from build123d import *

# Parameters (mm, degrees)
SKETCH1_W           = 133.35
SKETCH1_H           = 101.6
BOSS_EXTRUDE1_DEPTH = 3.175
SKETCH2_W           = 3.175
SKETCH2_H           = 12.192
SKETCH2_W_2         = 19.05
SKETCH2_H_2         = 6.35
BOSS_EXTRUDE2_DEPTH = 3.175
SKETCH3_W           = 19.05
SKETCH3_H           = 6.35
SKETCH3_H_2         = 6.604
CUT_EXTRUDE1_DEPTH  = 91.306287849


with BuildPart() as part:
    # Sketch1 → Boss-Extrude1 (new body)
    with BuildSketch(Plane(origin=(0, 0, 0), x_dir=(1, 0, 0), z_dir=(0, 1, 0))):
        Rectangle(SKETCH1_W, SKETCH1_H)
    extrude(amount=BOSS_EXTRUDE1_DEPTH)

    # Sketch2 → Boss-Extrude2 (add)
    with BuildSketch(Plane(origin=(0, 0, 0), x_dir=(-1, 0, 0), z_dir=(0, -1, 0))):
        with Locations((68.2625, -31.75)):
            Rectangle(SKETCH2_W, SKETCH2_H)
        with Locations((68.2625, -6.35)):
            Rectangle(SKETCH2_W, SKETCH2_H)
        with Locations((68.2625, 19.05)):
            Rectangle(SKETCH2_W, SKETCH2_H)
        with Locations((68.2625, 44.45)):
            Rectangle(SKETCH2_W, SKETCH2_H)
        with Locations((-68.2625, 44.45)):
            Rectangle(SKETCH2_W, SKETCH2_H)
        with Locations((-68.2625, 19.05)):
            Rectangle(SKETCH2_W, SKETCH2_H)
        with Locations((-68.2625, -6.35)):
            Rectangle(SKETCH2_W, SKETCH2_H)
        with Locations((-68.2625, -31.75)):
            Rectangle(SKETCH2_W, SKETCH2_H)
        with Locations((19.05, 53.975)):
            Rectangle(SKETCH2_W_2, SKETCH2_H_2)
        with Locations((57.15, 53.975)):
            Rectangle(SKETCH2_W_2, SKETCH2_H_2)
        with Locations((-19.05, 53.975)):
            Rectangle(SKETCH2_W_2, SKETCH2_H_2)
        with Locations((-57.15, 53.975)):
            Rectangle(SKETCH2_W_2, SKETCH2_H_2)
    extrude(amount=-BOSS_EXTRUDE2_DEPTH)

    # Sketch3 → Cut-Extrude1 (cut, through all)
    with BuildSketch(Plane(origin=(0, 0, 0), x_dir=(1, 0, 0), z_dir=(0, 1, 0))):
        with Locations((-57.15, 53.975)):
            Rectangle(SKETCH3_W, SKETCH3_H)
        with Locations((57.15, 53.848)):
            Rectangle(SKETCH3_W, SKETCH3_H_2)
    extrude(amount=CUT_EXTRUDE1_DEPTH, mode=Mode.SUBTRACT)


solid = part.part
Work out the finished part from the listing and answer in its coordinate system (mm). A direction names the side the tool comes from. Round coordinates to 2 decimals unless told otherwise and drop trailing zeros. Write each loop counter-clockwise with the first axis right and the second up, starting at its lowest first coordinate (ties: lowest second). Pieces come first, ordered by that corner, then holes.
1) A cutting plane is placed at A-A (z = 18.5). Give the vertices of the cut face in (x, y) (3 decimals), plus the area to 3 significant figures.
2) A tool of negligible diameter and unlimited length cuts with its end or side. For faces 4 (the flat face through (68, 2, 12.446)), 5 (the flat face through (-68, 2, 0.254)), 6 (the flat face through (-68, 2, -50.546)), from which of +Z, -Z, +X, -X, +Y, -Y can it reach the whole face along a straight path? Write none if from no direction.
3) Straight lines are drawn through the part: line 1 (Z direction, x = -7, y = 2.3); line 2 (X direction, y = 0.4, z = 23.5) (3 decimals); line 3 (Z direction, x = 56.5, y = 0.75). For each, find the intervals that lie inside material, in ascending order.
4) Given pin 1 Ø1 at (y, z) = (1.5, -7) entering from -X (3 decimals); pin 2 Ø1.6 at (y, z) = (1, -3.5) entering from +X (3 decimals); pin 3 Ø1.6 at (x, y) = (-69, 2) entering from +Z; pin 4 Ø6 at (x, z) = (-46.5, 7.5) entering from -Y, each flat-ended and moving along its own axis, determine where each tip first touches the part or whether it passes through.
5) The mould has two halves that part along Z. Classify faces 1 (the flat face through (-68, 2, 37.846)), 2 (the flat face through (28.575, 2, -54)), 3 (the flat face through (68, 2, 25.654)): pulls with the +Z half, pulls with the -Z half, needs draft (parallel to the pull), parting line crosses it, or undercut.
6) A cutting plane is placed at B-B (x = 33.5). Give the vertices of the cut face in (y, z) (3 decimals).
Completed:
1. outline: (-66.675, 0) - (66.675, 0) - (66.675, 3.175) - (-66.675, 3.175) - close
1. area: 423 mm2
2. face 4: +X, +Y, -Y
2. face 5: -X, +Y, -Y
2. face 6: -Z, -X, +Y, -Y
3. line 1: z = -50.8 to 50.8
3. line 2: x = -66.675 to 66.675
3. line 3: z = -50.55 to 50.8
4. pin 1: stops at x = -66.675
4. pin 2: stops at x = 66.675
4. pin 3: stops at z = 37.85
4. pin 4: stops at y = 0
5. face 1: pulls with the +Z half
5. face 2: needs draft
5. face 3: undercut
6. outline: (0, -50.8) - (3.175, -50.8) - (3.175, 50.8) - (0, 50.8) - close
